Input: part model. Units: mm. Frame: model coordinates. A direction names the side the tool comes from. Give positions to 0.01 mm unless a question says otherwise; leave off trailing zeros. Loops run counter-clockwise (first coordinate to the right, second up) from the corner with the lowest first, then second, coordinate; pieces in that order, holes last. Notation, with made-up numbers: M 27,-11.75 L 34,-11.75 A26 ccw 34,24.25 Z; hole C 10,70 d4. An arc over 180 degrees is marked long. Answer as a JSON object with one key per item and string values. Group by question number.
1) Section query C-C on z = 17. Return loops of the section in (x, y), plus the area to 3 significant figures.
2) Ray query, L1, parallel to Y at x = -40.5, z = 10; L2, parallel to X at y = 15.5, z = 22.75; L3, parallel to X at y = 15, z = 22. Return the intervals inside material, ascending.
3) Section query A-A on z = 5.5. Return loops of the section in (x, y).
4) Access query for faces 1 (the flat face through (45, 3, 4)), 2 (the flat face through (-0.1, 27.3, 10)), 3 (the flat face through (-0.2, 28.2, 13)). Directions: +Z, -Z, +X, -X, +Y, -Y. A direction counts if a zero-diameter tool reaches every point of the face in a straight line with its end or side. Return the directions, or none.
5) Section query B-B on x = 0. Return loops of the section in (y, z), plus the area to 3 significant figures.
6) Draft query along X for faces 4 (the cylindrical face through (44.61, 1.48, 4.31)), 5 (the flat face through (-42, 2, 12)), 6 (the cylindrical face through (-0.55, 24.994, 18.409)), 7 (the cylindrical face through (-0.648, 32.994, 5.423)). Return one class per face: +X half, -X half, draft (parallel to the pull), parting line (faces both ways), or undercut.
7) First-contact query: P1, Ø3, axis at x = -18, z = 15.5, coming from the -Y side; P2, Ø8, axis at y = 8, z = 5.5, coming from the -X side; P3, Ø2, axis at x = -29.5, z = 9.5, coming from the -Y side; P4, Ø5.5, axis at x = -41, z = 5.5, coming from the +Y side. Flat tips, straight axial feed; report the tip coordinate or a pass-through.
Autodesk Inventor part; units mm, degrees
ref_plane "YZ Plane" through (0, 0, 0) normal (1, 0, 0) x (0, 1, 0)
ref_plane "XZ Plane" through (0, 0, 0) normal (0, 1, 0) x (-1, 0, 0)
ref_plane "XY Plane" through (0, 0, 0) normal (0, 0, 1) x (1, 0, 0)
sketch "Sketch1" plane through (0, 0, 0) normal (0, 0, 1) x (1, 0, 0)
  circle A0 centre (0, 0) radius 30
  line L0 (-33, 0) -> (-48, 0)
  line L1 (-48, 0) -> (-48, 3)
  line L2 (-48, 3) -> (-35.4965, 3)
  arc A1 (-35.4965, 3) -> (-32.5384, 5.5) centre (-35.4965, 6) ccw
  line L3 (0, 35.372) -> (0, -34.8897)
  line L4 (33, 0) -> (48, 0)
  line L5 (48, 0) -> (48, 3)
  line L6 (48, 3) -> (35.4965, 3)
  arc A2 (32.5384, 5.5) -> (35.4965, 3) centre (35.4965, 6) ccw
  arc A3 (-33, 0) -> (33, 0) centre (0, 0) ccw
  arc A4 (32.5384, 5.5) -> (-32.5384, 5.5) centre (0, 0) ccw
  line L7 (33, 0) -> (30, 0)
  line L8 (-33, 0) -> (-30, 0)
  point P0 (-32.8634, 3)
  dimension "d0" = 60
  dimension "d4" = 15
  dimension "d5" = 3
  dimension "d6" = 3
extrude "Extrusion1" add sketch "Sketch1" along normal blind 13 contours A0 L3 A4 A2 L6 L5 L4 L7 | A0 L8 L0 L1 L2 A1 A4 L3
sketch "Sketch2" plane through (0, 0, 0) normal (0, 1, 0) x (-1, 0, 0)
  line L0 (-30, 0) -> (-30, 13) construction
  line L1 (-30, 0) -> (-33, 0) construction
  line L2 (-30, 0) -> (-48, 0) construction
  line L3 (-33, 0) -> (-33, 13) construction
  line L4 (-33, 13) -> (-28, 13) construction
  line L5 (-35.4965, 13) -> (-32.5384, 13) construction
  line L6 (-30, 13) -> (-28, 13)
  line L7 (-28, 13) -> (-28, 25)
  line L8 (-28, 25) -> (-25, 25)
  line L9 (-25, 25) -> (-25, 12)
  line L10 (-27, 10) -> (-30, 10)
  line L11 (-27, 10) -> (-25, 12)
  line L12 (-30, 10) -> (-30, 13)
  line L13 (0, -5) -> (0, 30)
  point P0 (0, 0)
  point P1 (-25, 10)
  dimension "d9" = 3
  dimension "d10" = 5
  dimension "d11" = 12
  dimension "d12" = 3
  dimension "d13" = 15
  dimension "d14" = 2
  dimension "d15" = 2
revolve "Revolution1" add sketch "Sketch2" angle 180 about axis through (0, 0, -10) along (0, 0, 1)
chamfer "Chamfer1" distance 2 angle 45 5 edges at (0, 33, 13) (-33.56, 3.7087, 13) (-41.7482, 3, 13) (33.56, 3.7087, 13) (41.7482, 3, 13)
sketch "Sketch3" plane through (-48, 0, 0) normal (0, -1, 0) x (1, 0, 0)
  line L0 (0, 0) -> (0, 13) construction
  line L1 (48, 0) -> (48, 25)
  line L2 (73, 25) -> (23, 25)
  line L3 (12.5035, 0) -> (0, 0)
  line L4 (6.2518, 0) -> (6.2518, 5.5) construction
  circle A0 centre (6.2518, 5.5) radius 3.1
  circle A1 centre (89.7482, 5.5) radius 3.1
  line L5 (0, 0) -> (0, 5.5) construction
  line L6 (0, 5.5) -> (6.2518, 5.5) construction
  dimension "d24" = 6.2
  dimension "d25" = 5.5
extrude "Extrusion2" cut sketch "Sketch3" against normal through all
properties part number "EXTRUSSOR-COUPLINGv2"
Output:
{
 "1": {"outline": "M -28,0 L -25,0 A25 cw 25,0 L 28,0 A28 ccw Z", "area": "250 mm^2"},
 "2": {"L1": "y = 0 to 3", "L2": "x = -23.32 to -19.62, 19.62 to 23.32", "L3": "x = -23.64 to -20, 20 to 23.64"},
 "3": {"outline": "M -48,0 L -44.85,0 L -44.85,3 L -48,3 Z; M -38.65,0 L -30,0 A30 cw 30,0 L 38.65,0 L 38.65,3 L 35.5,3 A3 cw 32.54,5.5 A33 ccw -32.54,5.5 A3 cw -35.5,3 L -38.65,3 Z; M 44.85,0 L 48,0 L 48,3 L 44.85,3 Z"},
 "4": {"face 1": "+Z, -Z, +X, +Y", "face 2": "-Z, -Y", "face 3": "+Z, +Y"},
 "5": {"outline": "M 25,12 L 27,10 L 30,10 L 30,0 L 33,0 L 33,11 L 31,13 L 28,13 L 28,25 L 25,25 Z", "area": "86.0 mm^2"},
 "6": {"face 4": "undercut", "face 5": "draft", "face 6": "undercut", "face 7": "parting line"},
 "7": {"P1": "stops at y = 15.64", "P2": "stops at x = -33.26", "P3": "stops at y = 0", "P4": "stops at y = 3"}
}
